Autodesk Inventor part; units mm, degrees
ref_plane "YZ Plane" through (0, 0, 0) normal (1, 0, 0) x (0, 1, 0)
ref_plane "XZ Plane" through (0, 0, 0) normal (0, 1, 0) x (-1, 0, 0)
ref_plane "XY Plane" through (0, 0, 0) normal (0, 0, 1) x (1, 0, 0)
ref_plane "Płaszczyzna konstrukcyjna1" through (33, 3, -33.6408) normal (0, 1, 0) x (0, 0, 1)
sketch "Szkic1" plane through (33, 3, -33.6408) normal (0, 1, 0) x (0, 0, 1)
  line L0 (33.6408, -11) -> (70.3592, -11)
  line L1 (33.6408, -33) -> (33.6408, -11)
  line L2 (33.6408, -11) -> (70.3592, -11)
  line L3 (70.3592, -11) -> (70.3592, -33)
  line L4 (70.3592, -33) -> (33.6408, -33)
  line L5 (33.6408, -33) -> (33.6408, -11)
extrude "Wyciągnięcie proste1" add sketch "Szkic1" against normal blind 3
sketch "Szkic2" plane through (33, 0, -33.6408) normal (0, -1, 0) x (1, 0, 0)
  line L0 (-11, 33.6408) -> (-33, 33.6408)
  line L1 (-33, 33.6408) -> (-33, 39.6408)
  line L2 (-33, 39.6408) -> (-11, 39.6408)
  line L3 (-11, 39.6408) -> (-11, 33.6408)
  line L4 (-33, 33.6408) -> (-11, 33.6408)
  line L5 (-11, 33.6408) -> (-11, 70.3592)
  line L6 (-33, 70.3592) -> (-33, 33.6408)
  dimension "d2" = 6
extrude "Wyciągnięcie proste2" add sketch "Szkic2" along normal blind 20
sketch "Szkic3" plane through (22, 3, 0) normal (0, 0, -1) x (-1, 0, 0)
  circle A0 centre (18.7, -6) radius 1.25
  circle A1 centre (3.3, -6) radius 1.25
  circle A2 centre (3.3, -20) radius 1.25
  circle A3 centre (18.7, -20) radius 1.25
  circle A4 centre (11, -13) radius 2.125
  circle A5 centre (18.7, -6) radius 1.5
  circle A6 centre (18.7, -20) radius 1.5
  circle A7 centre (3.3, -6) radius 1.5
  circle A8 centre (3.3, -20) radius 1.5
  point P0 (22, -3)
  dimension "d5" = 0.25
  dimension "d6" = 0.25
  dimension "d7" = 0.25
  dimension "d8" = 0.25
extrude "Wyciągnięcie proste3" cut sketch "Szkic3" against normal through all contours A0 | A1 | A2 | A3 | A4 | A5 | A6 | A7 | A8
sketch "Szkic4" plane through (33, 3, -33.6408) normal (0, 1, 0) x (1, 0, 0)
  line L0 (-33, -48.2408) -> (-22, -48.2408) construction
  line L1 (-22, -48.2408) -> (-11, -48.2408) construction
  line L2 (-11, -70.3592) -> (-11, -33.6408)
  line L3 (-33, -33.6408) -> (-33, -70.3592)
  line L4 (-11, -33.6408) -> (-33, -33.6408)
  line L5 (-22, -48.2408) -> (-22, -33.6408) construction
  line L6 (-22, -48.2408) -> (-22, -62.8408) construction
  line L7 (-11, -33.6408) -> (-33, -33.6408)
  line L8 (-33, -33.6408) -> (-33, -62.8408)
  line L9 (-33, -62.8408) -> (-11, -62.8408)
  line L10 (-11, -62.8408) -> (-11, -33.6408)
  point P0 (-11, -62.8408)
  dimension "d11" = 14.6
extrude "Wyciągnięcie proste4" cut sketch "Szkic4" against normal through all keep common part
sketch "Szkic6" plane through (33, 3, -33.6408) normal (0, 1, 0) x (1, 0, 0)
  line L0 (-11, -62.8408) -> (-33, -62.8408)
  line L1 (-11, -62.8408) -> (-11, -33.6408)
  line L2 (-11, -33.6408) -> (-33, -33.6408)
  line L3 (-33, -33.6408) -> (-33, -62.8408)
extrude "Wyciągnięcie proste5" add sketch "Szkic6" along normal blind 10.5
hole "Otwór3" at (11, 3, 14.6) direction (0, -1, 0) diameter 4.25 end through all both
sketch "Szkic7" plane through (33, 0, -33.6408) normal (0, -1, 0) x (1, 0, 0)
  circle A0 centre (-22, 48.2408) radius 2.125
  circle A1 centre (-22, 48.2408) radius 4.5
  point P0 (-33, 33.6408)
  dimension "d37" = 9
extrude "Wyciągnięcie proste6" cut sketch "Szkic7" against normal blind 12 contours A0 | A1
sketch "Szkic8" plane through (33, -20, -33.6408) normal (0, -1, 0) x (1, 0, 0)
  line L0 (-33, 33.6408) -> (-11, 33.6408)
  line L1 (-11, 33.6408) -> (-11, 39.6408)
  line L2 (-11, 39.6408) -> (-33, 39.6408)
  line L3 (-33, 39.6408) -> (-33, 33.6408)
extrude "Wyciągnięcie proste7" add sketch "Szkic8" along normal blind 18
mirror "Odbij1" about plane through (11, -38, 3) normal (0, -1, 0)
sketch "Szkic9" plane through (0, 0, 6) normal (0, 0, 1) x (1, 0, 0)
  circle A0 centre (11, -66) radius 2.125
  circle A1 centre (18.7, -73) radius 1.5
  circle A2 centre (3.3, -73) radius 1.5
  circle A3 centre (18.7, -59) radius 1.5
  circle A4 centre (3.3, -59) radius 1.5
  circle A5 centre (3.3, -17) radius 1.5
  circle A6 centre (18.7, -17) radius 1.5
  circle A7 centre (3.3, -3) radius 1.5
  circle A8 centre (18.7, -3) radius 1.5
  circle A9 centre (11, -10) radius 2.125
  line L0 (0, 0) -> (22, 0)
  line L1 (0, 0) -> (0, -76)
  line L2 (0, -76) -> (22, -76)
  line L3 (22, 0) -> (22, -76)
  circle A10 centre (11, -66) radius 2.125
  circle A11 centre (11, -66) radius 4.5
  circle A12 centre (11, -10) radius 4.5
  point P0 (0, 0)
  dimension "d42" = 9
  dimension "d43" = 9
extrude "Wyciągnięcie proste8" add sketch "Szkic9" along normal up to surface (23.2 mm away) contours L0 L3 L2 L1
sketch "Szkic11" plane through (0, 13.5, 29.2) normal (0, 0, 1) x (1, 0, 0)
  line L0 (6.5, -3) -> (15.5, -3)
  line L1 (15.5, -3) -> (15.5, -28)
  line L2 (15.5, -28) -> (6.5, -28)
  line L3 (6.5, -28) -> (6.5, -3)
  line L4 (6.5, -75) -> (15.5, -75)
  line L5 (15.5, -75) -> (15.5, -100)
  line L6 (15.5, -100) -> (6.5, -100)
  line L7 (6.5, -100) -> (6.5, -75)
  line L8 (0, 0) -> (0, -103) construction
  line L9 (0, 0) -> (6.5, -3) construction
  line L10 (15.5, -3) -> (22, 0) construction
  line L11 (0, 0) -> (22, 0) construction
  line L12 (0, -103) -> (22, -103) construction
  circle A0 centre (11, -23.5) radius 4.5
  circle A1 centre (11, -79.5) radius 4.5
  point P0 (0, -13.5)
  dimension "d48" = 3
  dimension "d51" = 3
extrude "Wyciągnięcie proste9" cut sketch "Szkic11" against normal blind 19.1
equation "\"d51\" = d48"
properties part number "wheel-adapter-front"
Could you check a few things on this model? Use its own coordinates, in mm. A direction names the side the tool comes from. Give positions to 0.01 mm unless a question says otherwise; leave off trailing zeros. Order: outer loops, then holes, each group sorted by start corner. A loop starts at its lowest first (then second) coordinate and runs counter-clockwise, first axis right, second up. Notation, with made-up numbers: (89.5, 32) - (97.5, 32) arc R24 ccw to (97.5, 67) - close; hole circle Ø6 at (78.5, 63). An arc over 180 degrees is marked (long way). One line per question, with ' | ' between items. Start each with the question number.
Item 1: I want a section at A-A on x = 18.7. Write out the boundary of the cut face in (y, z).
Item 2: I need wall thicknesses on probe 1 along X at (y, z) = (-73, 27); probe 2 along Y at (x, z) = (7, 18.5); probe 3 along X at (y, z) = (-17, 23.5). Which ranges of each line are inside material? Lowest first, please. Write a range as [from, to].
Item 3: I want a section at B-B on z = 2.25. Give the number of separate pieces and of enclosed holes in the cut face, then the cut area to 3 significant figures.
Item 4: Thinking about a two-plate mould opening in X: for faces 1 (the flat face through (11, -39, 29.2)), 2 (the flat face through (7, -63, 10.1)), 3 (the flat face through (14, -62, 10.1)), which applies, pulls with the +X half, pulls with the -X half, needs draft (parallel to the pull), parting line crosses it, or undercut?
Item 5: For faces 4 (the flat face through (8.7, -89.5, 14.4)), 5 (the flat face through (9, -88, 16)), 6 (the flat face through (10.1, -7.9, 6)), 7 (the flat face through (11, -37, 0)), 8 (the cylindrical face through (10.186, -88.74, 16.563)), which set-ups out of +Z, -Z, +X, -X, +Y, -Y let a thin tool reach every point of the face, with its end or its side?
Item 6: I want a section at C-C on y = -73. Write out the boundary of the cut face in (x, z).
Item 7: I'm going to push flat-ended pins straight in: pin 1 Ø1.8 at (x, y) = (18.7, -3) entering from -Z; pin 2 Ø3.5 at (x, y) = (18.7, -59) entering from +Z; pin 3 Ø2.5 at (x, z) = (11, 14.6) entering from -Y. Where does each tip first touch, or does it pass through?
Verdict:
1) outline: (-89.5, 0) - (-74.5, 0) - (-74.5, 29.2) - (-89.5, 29.2) - close; (-71.5, 0) - (-60.5, 0) - (-60.5, 29.2) - (-71.5, 29.2) - close; (-57.5, 0) - (-18.5, 0) - (-18.5, 29.2) - (-57.5, 29.2) - close; (-15.5, 0) - (-4.5, 0) - (-4.5, 29.2) - (-15.5, 29.2) - close; (-1.5, 0) - (13.5, 0) - (13.5, 29.2) - (-1.5, 29.2) - close
2) probe 1: [0, 1.8], [4.8, 6.5], [15.5, 17.2], [20.2, 22] | probe 2: [-89.5, -86.5], [-61.5, -14.5], [10.5, 13.5] | probe 3: [0, 1.8], [4.8, 17.2], [20.2, 22]
3) separate pieces: 1 | enclosed holes: 10 | area: 2,180 mm^2
4) face 1: needs draft | face 2: undercut | face 3: undercut
5) face 4: +Z, -Z, +X, -X, -Y | face 5: none | face 6: +Z | face 7: -Z, +X, -X, +Y, -Y | face 8: -Y
6) outline: (0, 0) - (1.8, 0) - (1.8, 29.2) - (0, 29.2) - close; (4.8, 0) - (17.2, 0) - (17.2, 29.2) - (15.5, 29.2) - (15.5, 10.1) - (6.5, 10.1) - (6.5, 29.2) - (4.8, 29.2) - close; (20.2, 0) - (22, 0) - (22, 29.2) - (20.2, 29.2) - close
7) pin 1: through | pin 2: z = 29.2 | pin 3: y = -61.5
